from build123d import *

# Parameters (mm, degrees)
EXTRUDE1_DEPTH     = 50.8
CUT_EXTRUDE1_DEPTH = 9.525
SKETCH3_R          = 7.9375
CUT_EXTRUDE2_DEPTH = 163.175685145
SKETCH4_W          = 50.8
SKETCH4_H          = 50.8
CUT_EXTRUDE3_DEPTH = 3.175
SKETCH5_R          = 2.38125
CUT_EXTRUDE4_DEPTH = 15.875
CUT_EXTRUDE5_START = -15.875
SKETCH6_R          = 2.38125
CUT_EXTRUDE5_DEPTH = 15.875
SKETCH7_R          = 3.175
CUT_EXTRUDE6_DEPTH = 163.175685145
SKETCH8_R          = 5.08
CUT_EXTRUDE7_DEPTH = 6.35
CUT_EXTRUDE8_DEPTH = 163.175685145
EXTRUDE2_DEPTH     = 50.8


with BuildPart() as part:
    # Sketch1 → Extrude1 (new body)
    with BuildSketch(Plane.XY):
        Polygon((0, 0), (-5.260512242, 12.7), (153.489487758, 12.7), (153.489487758, 0), align=None)
    extrude(amount=EXTRUDE1_DEPTH)

    # Sketch2 → Cut-Extrude1 (cut)
    with BuildSketch(Plane.XZ):
        with BuildLine():
            Line((19.05, 41.275), (63.5, 41.275))
            ThreePointArc((63.5, 41.275), (67.990128061, 39.415128061), (69.85, 34.925))
            Line((69.85, 34.925), (69.85, 15.875))
            ThreePointArc((69.85, 15.875), (67.990128061, 11.384871939), (63.5, 9.525))
            Line((63.5, 9.525), (19.05, 9.525))
            ThreePointArc((19.05, 9.525), (14.559871939, 11.384871939), (12.7, 15.875))
            Line((12.7, 15.875), (12.7, 34.925))
            ThreePointArc((12.7, 34.925), (14.559871939, 39.415128061), (19.05, 41.275))
        make_face()
    extrude(amount=-CUT_EXTRUDE1_DEPTH, mode=Mode.SUBTRACT)

    # Sketch3 → Cut-Extrude2 (cut, through all)
    with BuildSketch(Plane.XZ):
        with Locations((109.039487758, 25.4)):
            Circle(SKETCH3_R)
    extrude(amount=-CUT_EXTRUDE2_DEPTH, mode=Mode.SUBTRACT)

    # Sketch4 → Cut-Extrude3 (cut)
    with BuildSketch(Plane.XZ):
        with Locations((109.039487758, 25.4)):
            Rectangle(SKETCH4_W, SKETCH4_H)
    extrude(amount=-CUT_EXTRUDE3_DEPTH, mode=Mode.SUBTRACT)

    # Sketch5 → Cut-Extrude4 (cut)
    with BuildSketch(Plane.XY.offset(50.8)):
        with Locations((7.439487758, 6.35)):
            Circle(SKETCH5_R)
    extrude(amount=-CUT_EXTRUDE4_DEPTH, mode=Mode.SUBTRACT)

    # Sketch6 → Cut-Extrude5 (cut)
    with BuildSketch(Plane(origin=(0, 0, 0), x_dir=(-1, 0, 0), z_dir=(0, 0, -1)).offset(CUT_EXTRUDE5_START)):
        with Locations(Location((-7.439487758, 6.35, 0), (0, 0, 180))):
            Circle(SKETCH6_R)
    extrude(amount=CUT_EXTRUDE5_DEPTH, mode=Mode.SUBTRACT)

    # Sketch7 → Cut-Extrude6 (cut, through all)
    with BuildSketch(Plane(origin=(0, 12.7, 0), x_dir=(-1, 0, 0), z_dir=(0, 1, 0))):
        with Locations(Location((-147.139487758, 9.525, 0), (0, 0, 90))):
            Circle(SKETCH7_R)
        with Locations(Location((-147.139487758, 41.275, 0), (0, 0, 90))):
            Circle(SKETCH7_R)
    extrude(amount=-CUT_EXTRUDE6_DEPTH, mode=Mode.SUBTRACT)

    # Sketch8 → Cut-Extrude7 (cut)
    with BuildSketch(Plane(origin=(0, 12.7, 0), x_dir=(-1, 0, 0), z_dir=(0, 1, 0))):
        with Locations(Location((-147.139487758, 9.525, 0), (0, 0, 90))):
            Circle(SKETCH8_R)
        with Locations(Location((-147.139487758, 41.275, 0), (0, 0, 90))):
            Circle(SKETCH8_R)
    extrude(amount=-CUT_EXTRUDE7_DEPTH, mode=Mode.SUBTRACT)

    # Sketch9 → Cut-Extrude8 (cut, through all)
    with BuildSketch(Plane.XY.offset(50.8)):
        with BuildLine():
            Line((5.260512242, 12.7), (-5.260512242, 12.7))
            Line((-5.260512242, 12.7), (-4.45964694, 10.766540126))
            ThreePointArc((-4.45964694, 10.766540126), (0.305218063, 12.211946122), (5.260512242, 12.7))
        make_face()
    extrude(amount=-CUT_EXTRUDE8_DEPTH, mode=Mode.SUBTRACT)

    # Sketch10 → Extrude2 (add)
    with BuildSketch(Plane.XY.offset(50.8)):
        with BuildLine():
            Line((0, 0), (0.400432651, -0.966729937))
            ThreePointArc((0.400432651, -0.966729937), (2.782865153, -0.244026939), (5.260512242, 0))
            Line((5.260512242, 0), (0, 0))
        make_face()
    extrude(amount=-EXTRUDE2_DEPTH)


solid = part.part
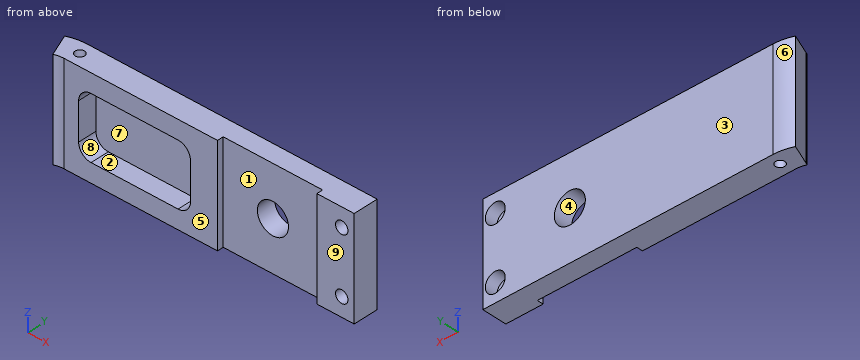
Geometry: final body of the model. Coordinates: model frame, mm. Face numbers are marked on the shaded views. A direction names the side the tool comes from. Coordinates: 2 decimals unless noted, no trailing zeros. Loops run counter-clockwise (first coordinate to the right, second up) from the corner with the lowest first, then second, coordinate; pieces in that order, holes last. Notation, with made-up numbers: M 51,-31 L 94,-31 A27 cw 94,-14 Z; hole C 22.5,73.25 d9. An arc over 180 degrees is marked long. One line per item, written item: value. Start each with the question number.
1) Cut plane D-D (z = 19.5). Return loops of the section in (x, y) (3 decimals), then the cut area to 3 significant figures.
2) Draft query along X for the marked faces 6, 7, 8 and 9. Return one class per face: released by +X, released by -X, zero draft, split by the parting line, or undercut.
3) Pin query (flat end, axial travel): P1, Ø9.5, axis at x = 144, z = 25, coming from the -Y side; P2, Ø9, axis at x = 147.14, z = 41.28, coming from the +Y side; P3, Ø1.5, axis at y = 1.5, z = 13.5, coming from the -X side. Return the tip coordinate at first contact, or that it passes through.
4) Material intervals for L1, parallel to Z at x = 23, y = 3.75 (3 decimals); L2, parallel to X at y = 7.25, z = 10.5; L3, parallel to X at y = 7.25, z = 40.5, sorted ascending. Write a range as from..to.
5) Cut plane C-C (x = 111). Return loops of the section in (y, z) (3 decimals), then the cut area to 3 significant figures.
6) Reachability of the marked faces 1, 2, 3, 4 and 5 from +Z, -Z, +X, -X, +Y, -Y: full face, straight path, thin tool, end or side. Return the list, or none.
7) Cut plane B-B (x = 30). Return loops of the section in (y, z) (3 decimals).
8) Cut plane A-A (z = 25.4). Return loops of the section in (x, y) (3 decimals), then the cut area to 3 significant figures.
Evaluation:
1. outline: M -4.46,10.767 L 0.4,-0.967 A12.7 cw 5.261,0 L 12.7,0 L 12.7,9.525 L 69.85,9.525 L 69.85,0 L 83.639,0 L 83.639,3.175 L 103.73,3.175 L 103.73,12.7 L 5.261,12.7 A25.4 ccw Z; M 114.349,3.175 L 134.439,3.175 L 134.439,0 L 153.489,0 L 153.489,12.7 L 114.349,12.7 Z
1. area: 1,170 mm^2
2. face 6: released by -X
2. face 7: undercut
2. face 8: undercut
2. face 9: zero draft
3. P1: y = 0
3. P2: y = 6.35
3. P3: x = -0.93
4. L1: 0..9.525, 41.275..50.8
4. L2: -3..5.23, 9.64..15.67, 66.88..142.15, 152.13..153.49
4. L3: -3..5.23, 9.64..16.01, 66.54..142.12, 152.16..153.49
5. outline: M 3.175,0 L 12.7,0 L 12.7,17.708 L 3.175,17.708 Z; M 3.175,33.092 L 12.7,33.092 L 12.7,50.8 L 3.175,50.8 Z
5. area: 337 mm^2
6. face 1: +Z, -Z, -Y
6. face 2: -Y
6. face 3: +Z, -Z, +X, -X, +Y
6. face 4: +Y, -Y
6. face 5: +Z, -Z, +X, -Y
7. outline: M 0,0 L 12.7,0 L 12.7,50.8 L 0,50.8 L 0,41.275 L 9.525,41.275 L 9.525,9.525 L 0,9.525 Z
8. outline: M -4.46,10.767 L 0.4,-0.967 A12.7 cw 5.261,0 L 12.7,0 L 12.7,9.525 L 69.85,9.525 L 69.85,0 L 83.639,0 L 83.639,3.175 L 101.102,3.175 L 101.102,12.7 L 5.261,12.7 A25.4 ccw Z; M 116.977,3.175 L 134.439,3.175 L 134.439,0 L 153.489,0 L 153.489,12.7 L 116.977,12.7 Z
8. area: 1,120 mm^2
